Geometry: final body of the model. Coordinates: model frame, mm. Coordinates: 2 decimals unless noted, no trailing zeros. Order: outer loops, then holes, each group sorted by start corner. A loop starts at its lowest first (then second) coordinate and runs counter-clockwise, first axis right, second up. Notation, with made-up numbers: (-24.75, 70.25) - (-0.75, 70.25) arc R20 ccw to (-0.75, 86.25) - close; hole circle Ø7 at (-4.5, 86). An arc over 180 degrees is marked (long way). Use a Markdown table: item, result. Add a question column.
```python
from build123d import *

# Parameters (mm, degrees)
F0_R     = 3.245174
F0_W     = 7.62
F0_H     = 10.16
F0_H_2   = 12.7
F1_DEPTH = 4.1275
F0_W_2   = 346.71
F0_H_3   = 5.715
F2_DEPTH = 3.175


with BuildPart() as f1:
    # F0 (on Front) → F1 (new body, symmetric)
    with BuildSketch(Plane.XZ):
        Polygon((173.355, 121.285), (-173.355, 121.285), (-173.355, -121.285), (173.355, -121.285), (173.355, -111.125), (173.355, -65.0875), (173.355, -52.3875), (173.355, -6.35), (173.355, 6.35), (173.355, 52.3875), (173.355, 65.0875), (173.355, 111.125), align=None)
        with Locations((-86.6902, -116.205)):
            Circle(F0_R, mode=Mode.SUBTRACT)
        with Locations((0, -116.205)):
            Circle(F0_R, mode=Mode.SUBTRACT)
        with Locations((86.6648, -116.205)):
            Circle(F0_R, mode=Mode.SUBTRACT)
        with Locations((-0.0254, 116.205)):
            Circle(F0_R, mode=Mode.SUBTRACT)
        with Locations((86.6648, 116.205)):
            Circle(F0_R, mode=Mode.SUBTRACT)
        with Locations((177.165, 116.205)):
            Rectangle(F0_W, F0_H)
        with Locations((177.165, 58.7375)):
            Rectangle(F0_W, F0_H_2)
        with Locations((177.165, 0)):
            Rectangle(F0_W, F0_H_2)
        with Locations((177.165, -58.7375)):
            Rectangle(F0_W, F0_H_2)
        with Locations((177.165, -116.205)):
            Rectangle(F0_W, F0_H)
    extrude(amount=F1_DEPTH, both=True)

    # F0 (on Front) → F2 (join, symmetric)
    with BuildSketch(Plane.XZ):
        with Locations((0, 124.1425)):
            Rectangle(F0_W_2, F0_H_3)
        with Locations((0, -124.1425)):
            Rectangle(F0_W_2, F0_H_3)
    extrude(amount=F2_DEPTH, both=True)


solid = f1.part
```
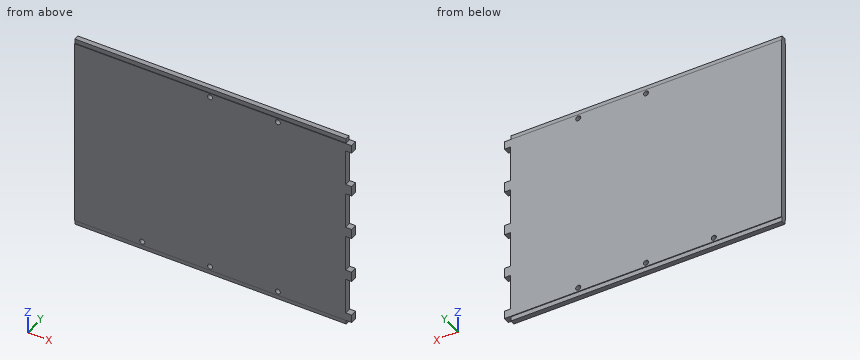
1) Section B-B (z = -14.5). Return loops of the section in (x, y) (1 decimal).
2) Pin query (flat end, axial travel): pin 1 (2.5 mm diameter, centred on x = 178.5, y = -1, fed in from +Z) (3 decimals); pin 2 (6.5 mm diameter, centred on x = 31.5, z = -125, fed in from +Y) (3 decimals); pin 3 (4 mm diameter, centred on x = 175.5, y = 0, fed in from -Z) (3 decimals). Return the tip coordinate at first contact, or that it passes through.
3) Ray query, line 1 along Z through (x, y) = (0, 2); line 2 along X through (y, z) = (-1.5, 37) (3 decimals); line 3 along Z through (x, y) = (62, -3.5) (3 decimals). Return the intervals inside material, ascending.
4) Section A-A (y = -1.75). Give the number of separate pieces and of enclosed holes in the cut face, then the cut area to 3 significant figures.
Values follow:
| question | item | result |
|---|---|---|
| 1 | outline | (-173.4, -4.1) - (173.4, -4.1) - (173.4, 4.1) - (-173.4, 4.1) - close |
| 2 | pin 1 | stops at z = 121.285 |
| 2 | pin 2 | stops at y = 3.175 |
| 2 | pin 3 | stops at z = -121.285 |
| 3 | line 1 | z = -127 to -119.45, -112.96 to 112.96, 119.45 to 127 |
| 3 | line 2 | x = -173.355 to 173.355 |
| 3 | line 3 | z = -121.285 to 121.285 |
| 4 | separate pieces | 1 |
| 4 | enclosed holes | 5 |
| 4 | area | 88,300 mm² |
